from build123d import *

# Parameters (mm, degrees)
SKETCH_1_W          = 134
SKETCH_1_H          = 80
EXTRUDE_352_DEPTH   = 24
FILLET_1_R          = 3
SHELL_1_T           = -2
SKETCH_2_W          = 50
SKETCH_2_H          = 42
SKETCH_2_W_2        = 10
SKETCH_2_H_2        = 10
CUT_EXTRUDE_1_DEPTH = 2
SKETCH_3_W          = 8
SKETCH_3_H          = 12
SKETCH_3_R          = 2
EXTRUDE_1169_DEPTH  = 2
SKETCH_4_W          = 8
SKETCH_4_H          = 2
EXTRUDE_3_DEPTH     = 8
SKETCH_5_W          = 8
SKETCH_5_H          = 2
EXTRUDE_4_DEPTH     = 8
CHAMFER_1_SIZE      = 8
SKETCH_6_W          = 10
SKETCH_6_H          = 2
EXTRUDE_5_DEPTH     = 4


with BuildPart() as part:
    # Эскиз1 → Extrude 352 (new body)
    with BuildSketch(Plane(origin=(0, 0, 0), x_dir=(1, 0, 0), z_dir=(0, 1, 0))):
        Rectangle(SKETCH_1_W, SKETCH_1_H)
    extrude(amount=EXTRUDE_352_DEPTH)

    # Скругление1
    fillet_1_edges = [part.edges().sort_by_distance(p)[0] for p in [
        (67, 24, 0),
        (0, 24, -40),
        (-67, 24, 0),
        (0, 24, 40),
        (-67, 12, -40),
        (67, 12, -40),
        (67, 12, 40),
        (-67, 12, 40),
    ]]
    fillet(fillet_1_edges, radius=FILLET_1_R)

    # Оболочка1
    shell_1_openings = [part.faces().sort_by_distance(p)[0] for p in [
        (0, 0, 0),
    ]]
    offset(amount=SHELL_1_T, openings=shell_1_openings, kind=Kind.INTERSECTION)

    # Эскиз2 → Вырез-Вытянуть1 (cut)
    with BuildSketch(Plane(origin=(0, 24, 0), x_dir=(1, 0, 0), z_dir=(0, 1, 0))):
        with Locations((18.5, 0.5)):
            Rectangle(SKETCH_2_W, SKETCH_2_H)
        with Locations((-50.5, 22.5)):
            Rectangle(SKETCH_2_W_2, SKETCH_2_H_2)
    extrude(amount=-CUT_EXTRUDE_1_DEPTH, mode=Mode.SUBTRACT)

    # Эскиз3 → Extrude 1169 (add)
    # profile 1 of 2: a face of its own
    with BuildSketch(Plane(origin=(0, 0, 0), x_dir=(1, 0, 0), z_dir=(0, 1, 0))):
        with Locations((-71, 0)):
            Rectangle(SKETCH_3_W, SKETCH_3_H)
        with Locations(Location((-71, 0, 0), (0, 0, 270))):
            Circle(SKETCH_3_R, mode=Mode.SUBTRACT)
    # profile 2 of 2: a face of its own
    with BuildSketch(Plane(origin=(0, 0, 0), x_dir=(1, 0, 0), z_dir=(0, 1, 0))):
        with Locations((71, 0)):
            Rectangle(SKETCH_3_W, SKETCH_3_H)
        with Locations(Location((71, 0, 0), (0, 0, 270))):
            Circle(SKETCH_3_R, mode=Mode.SUBTRACT)
    extrude(amount=EXTRUDE_1169_DEPTH)

    # Эскиз4 → Бобышка-Вытянуть3 (add)
    with BuildSketch(Plane(origin=(0, 2, 0), x_dir=(1, 0, 0), z_dir=(0, 1, 0))):
        with Locations((-71, 5)):
            Rectangle(SKETCH_4_W, SKETCH_4_H)
        with Locations((-71, -5)):
            Rectangle(SKETCH_4_W, SKETCH_4_H)
    extrude(amount=EXTRUDE_3_DEPTH)

    # Эскиз5 → Бобышка-Вытянуть4 (add)
    with BuildSketch(Plane(origin=(0, 2, 0), x_dir=(1, 0, 0), z_dir=(0, 1, 0))):
        with Locations((71, 5)):
            Rectangle(SKETCH_5_W, SKETCH_5_H)
        with Locations((71, -5)):
            Rectangle(SKETCH_5_W, SKETCH_5_H)
    extrude(amount=EXTRUDE_4_DEPTH)

    # Фаска1
    chamfer_1_edges = [part.edges().sort_by_distance(p)[0] for p in [
        (75, 10, 5),
        (75, 10, -5),
        (-75, 10, 5),
        (-75, 10, -5),
    ]]
    chamfer(chamfer_1_edges, length=CHAMFER_1_SIZE - 0.0001)  # a hair under: the kernel refuses the full size

    # Эскиз6 → Бобышка-Вытянуть5 (add)
    with BuildSketch(Plane.XZ.offset(-22)):
        with Locations((-50.5, -14)):
            Rectangle(SKETCH_6_W, SKETCH_6_H)
    extrude(amount=EXTRUDE_5_DEPTH)


solid = part.part
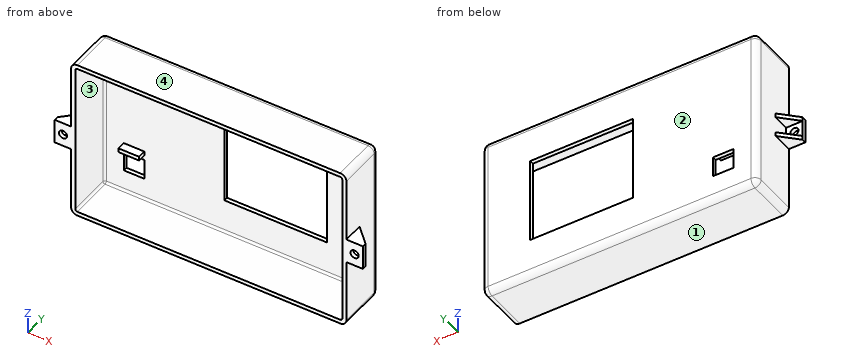
Build history of the part. All positions in model axes, mm. Face numbers are marked on the shaded views. Round coordinates to 2 decimals unless told otherwise and drop trailing zeros. Loops run counter-clockwise (first coordinate to the right, second up) from the corner with the lowest first, then second, coordinate; pieces in that order, holes last. Notation, with made-up numbers: (-14.5, 80) -> (25.5, 80) arc R26 cw to (25.5, 116) -> close; hole circle Ø10 at (51, 74). An arc over 180 degrees is marked (long way). Answer in a Markdown table with one row per item.
Item 1: Saw through at D-D (z = 26). Write the cut outline in (x, y), and give its area (3 significant figures).
Answers below:
| item | result |
|---|---|
| outline | (-67, 0) -> (-65, 0) -> (-65, 21) arc R1 cw to (-64, 22) -> (64, 22) arc R1 cw to (65, 21) -> (65, 0) -> (67, 0) -> (67, 21) arc R3 ccw to (64, 24) -> (-64, 24) arc R3 ccw to (-67, 21) -> close |
| area | 353 mm² |
Item 2: Pin check, flat tips, straight feed: pin 1 (6.5 mm diameter, centred on y = 12.5, z = -7.5, fed in from -X); pin 2 (8 mm diameter, centred on y = 4, z = 23, fed in from +X); pin 3 (10 mm diameter, centred on y = 11.5, z = -2, fed in from -X). Stop position of each tip, or through.
Answers below:
| item | result |
|---|---|
| pin 1 | stops at x = -67.38 |
| pin 2 | stops at x = 67 |
| pin 3 | stops at x = -70.08 |
Item 3: Saw through at B-B (y = 13.5). Write the cut outline in (x, z).
Answers below:
| item | result |
|---|---|
| outline | (-67, -37) arc R3 ccw to (-64, -40) -> (64, -40) arc R3 ccw to (67, -37) -> (67, 37) arc R3 ccw to (64, 40) -> (-64, 40) arc R3 ccw to (-67, 37) -> close; hole (-65, -37) arc R1 ccw to (-64, -38) -> (64, -38) arc R1 ccw to (65, -37) -> (65, 37) arc R1 ccw to (64, 38) -> (-64, 38) arc R1 ccw to (-65, 37) -> close |
Item 4: Drill centre lines: L1, parallel to X at y = 0.8, z = 0; L2, parallel to Z at x = -62, y = 11; L3, parallel to X at y = 2, z = 10. Where is each one in solid material? Low to high. Write a range as [from, to].
Answers below:
| item | result |
|---|---|
| L1 | x = [-75, -73], [-69, -65], [65, 69], [73, 75] |
| L2 | z = [-40, -38], [38, 40] |
| L3 | x = [-67, -65], [65, 67] |
Item 5: Mould opens along Z. For the marked faces 1, 2, 3 and 4 say: +Z half, -Z half, draft (parallel to the pull), parting line (faces both ways), or undercut.
Answers below:
| item | result |
|---|---|
| face 1 | -Z half |
| face 2 | draft |
| face 3 | undercut |
| face 4 | +Z half |
Item 6: Saw through at C-C (x = 11.5). Write the cut outline in (y, z), and give its area (3 significant figures).
Answers below:
| item | result |
|---|---|
| outline | (0, -40) -> (21, -40) arc R3 ccw to (24, -37) -> (24, -21.5) -> (22, -21.5) -> (22, -37) arc R1 cw to (21, -38) -> (0, -38) -> close; (0, 38) -> (21, 38) arc R1 cw to (22, 37) -> (22, 20.5) -> (24, 20.5) -> (24, 37) arc R3 ccw to (21, 40) -> (0, 40) -> close |
| area | 161 mm² |
Item 7: Saw through at A-A (z = 0). Write the cut outline in (x, y).
Answers below:
| item | result |
|---|---|
| outline | (-75, 0) -> (-73, 0) -> (-73, 2) -> (-75, 2) -> close; (-69, 0) -> (-65, 0) -> (-65, 21) arc R1 cw to (-64, 22) -> (-6.5, 22) -> (-6.5, 24) -> (-64, 24) arc R3 ccw to (-67, 21) -> (-67, 2) -> (-69, 2) -> close; (43.5, 22) -> (64, 22) arc R1 cw to (65, 21) -> (65, 0) -> (69, 0) -> (69, 2) -> (67, 2) -> (67, 21) arc R3 ccw to (64, 24) -> (43.5, 24) -> close; (73, 0) -> (75, 0) -> (75, 2) -> (73, 2) -> close |
